Here's how the part is built. I have some questions about the finished solid (model axes, mm). Round coordinates to 2 decimals unless told otherwise and drop trailing zeros. Order: outer loops, then holes, each group sorted by start corner. A loop starts at its lowest first (then second) coordinate and runs counter-clockwise, first axis right, second up. Notation, with made-up numbers: (35.25, 45) - (78.25, 45) arc R19 cw to (78.25, 58) - close; hole circle Ø9 at (31.5, -24.75). An arc over 180 degrees is marked (long way). Answer as a JSON object with one key per item and string values.
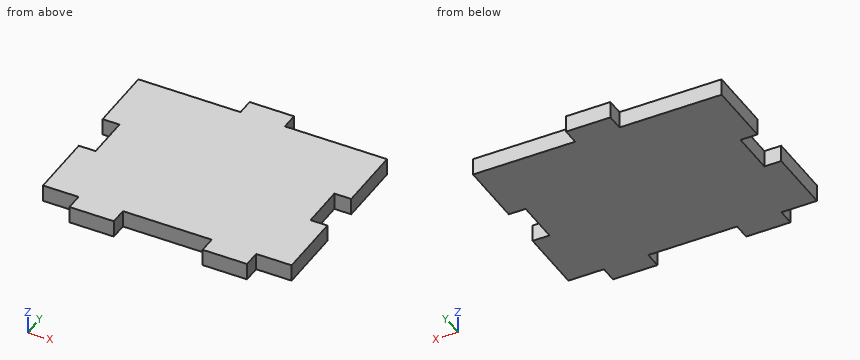
Autodesk Inventor part; units mm, degrees
ref_plane "YZ Plane" through (0, 0, 0) normal (1, 0, 0) x (0, 1, 0)
ref_plane "XZ Plane" through (0, 0, 0) normal (0, 1, 0) x (-1, 0, 0)
ref_plane "XY Plane" through (0, 0, 0) normal (0, 0, 1) x (1, 0, 0)
sketch "Sketch1" plane through (0, 0, 0) normal (0, 0, 1) x (1, 0, 0)
  line L0 (-34.925, 0) -> (34.925, 0)
  line L1 (-34.925, 4.826) -> (34.925, 4.826)
  line L2 (-25.4, 0) -> (-12.7, 0)
  line L3 (-25.4, 0) -> (-25.4, 4.826)
  line L4 (-12.7, 4.826) -> (-25.4, 4.826)
  line L5 (-12.7, 0) -> (-12.7, 4.826)
  line L6 (12.7, 0) -> (25.4, 0)
  line L7 (12.7, 0) -> (12.7, 4.826)
  line L8 (25.4, 4.826) -> (12.7, 4.826)
  line L9 (25.4, 0) -> (25.4, 4.826)
  line L10 (-34.925, 0) -> (-34.925, 4.826)
  line L11 (34.925, 4.826) -> (34.925, 0)
  point P0 (0, 0)
ref_plane "Work Plane1" through (-12.7, 0, -7.366) normal (0, 0, 1) x (1, 0, 0)
sketch "Sketch2" plane through (-12.7, 0, -7.366) normal (0, 0, 1) x (1, 0, 0)
  line L0 (0, 0) -> (-12.7, 0)
  line L1 (0, 0) -> (0, 4.826)
  line L2 (-12.7, 4.826) -> (0, 4.826)
  line L3 (-12.7, 0) -> (-12.7, 4.826)
  line L4 (-12.7, 0) -> (0, 0)
  line L5 (0, 0) -> (0, 4.826)
  line L6 (-12.7, 4.826) -> (-12.7, 0)
  line L7 (38.1, 0) -> (25.4, 0)
  line L8 (38.1, 0) -> (38.1, 4.826)
  line L9 (25.4, 4.826) -> (38.1, 4.826)
  line L10 (25.4, 0) -> (25.4, 4.826)
  line L11 (25.4, 0) -> (38.1, 0)
  line L12 (38.1, 0) -> (38.1, 4.826)
  line L13 (25.4, 4.826) -> (25.4, 0)
  line L14 (-18.034, 0) -> (-22.86, 0)
  line L15 (-18.034, 0) -> (-18.034, 4.826)
  line L16 (-22.86, 4.826) -> (-18.034, 4.826)
  line L17 (-22.86, 0) -> (-22.86, 4.826)
  line L18 (43.434, 0) -> (48.26, 0)
  line L19 (43.434, 0) -> (43.434, 4.826)
  line L20 (48.26, 4.826) -> (43.434, 4.826)
  line L21 (48.26, 0) -> (48.26, 4.826)
  line L22 (48.26, 55.626) -> (-22.86, 55.626)
  line L23 (-22.86, 36.576) -> (-18.034, 36.576)
  line L24 (-18.034, 36.576) -> (-18.034, 23.876)
  line L25 (-18.034, 23.876) -> (-22.86, 23.876)
  line L26 (48.26, 36.576) -> (43.434, 36.576)
  line L27 (43.434, 36.576) -> (43.434, 23.876)
  line L28 (43.434, 23.876) -> (48.26, 23.876)
  line L29 (-22.86, 55.626) -> (-22.86, 36.576)
  line L30 (-22.86, 23.876) -> (-22.86, 4.826)
  line L31 (48.26, 4.826) -> (48.26, 23.876)
  line L32 (48.26, 36.576) -> (48.26, 55.626)
  line L33 (-22.86, 4.826) -> (-12.7, 4.826)
  line L34 (0, 4.826) -> (25.4, 4.826)
  line L35 (38.1, 4.826) -> (48.26, 4.826)
  point P0 (12.7, 0)
  dimension "d0" = 50.8
  dimension "d2" = 12.7
  dimension "d5" = 4.826
  dimension "d13" = 19.05
  dimension "d14" = 19.05
  dimension "d15" = 12.7
extrude "Extrusion1" add sketch "Sketch2" along normal blind 4.826 contours L0 L3 L2 L1 | L2 L33 L16 L30 L25 L24 L23 L29 L22 L32 L26 L27 L28 L31 L20 L35 L9 L34 | L9 L8 L7 L10
sketch "Sketch3" plane through (-12.7, 0, -2.54) normal (0, 0, 1) x (1, 0, 0)
  line L0 (48.26, 55.626) -> (-22.86, 55.626)
  line L1 (-22.86, 55.626) -> (-22.86, 36.576)
  line L2 (48.26, 55.626) -> (-22.86, 55.626)
  line L3 (6.35, 55.626) -> (19.05, 55.626)
  line L4 (19.05, 55.626) -> (19.05, 60.452)
  line L5 (19.05, 60.452) -> (6.35, 60.452)
  line L6 (6.35, 60.452) -> (6.35, 55.626)
  point P0 (12.7, 0)
  dimension "d8" = 12.7
  dimension "d9" = 4.826
  dimension "d10" = 29.21
extrude "Extrusion2" add sketch "Sketch3" against normal blind 4.826
properties part number "sideL"
1. Imagine slicing it at B-B (x = -15.5). List the corners of the cut face in (y, z) for me.
Responses:
{"outline": "(0, -7.37) - (55.63, -7.37) - (55.63, -2.54) - (0, -2.54) - close"}
2. Imagine slicing it at C-C (y = 34.5). List the corners of the cut face in (x, z) for me.
Responses:
{"outline": "(-30.73, -7.37) - (30.73, -7.37) - (30.73, -2.54) - (-30.73, -2.54) - close"}
3. If I drill on L1, parallel to X at y = 4.5, z = -4.7; L2, parallel to Y at x = -17, z = -4.45; L3, parallel to X at y = 25, z = -4.75, over which ranges is the centre line in solid material (lowest first)? Write a range as [from, to].
Responses:
{"L1": "[-25.4, -12.7], [12.7, 25.4]", "L2": "[0, 55.63]", "L3": "[-30.73, 30.73]"}
4. For P1, Ø1.4, axis at y = 58.5, z = -5, coming from the +X side; P2, Ø2.5, axis at y = 2, z = -6, coming from the -X side; P3, Ø2.5, axis at y = 1.5, z = -4.5, coming from the +X side, each with a flat end and sliding along its axis, tell me the tip position at first contact or that it passes through.
Responses:
{"P1": "x = 6.35", "P2": "x = -25.4", "P3": "x = 25.4"}
5. Imagine slicing it at A-A (z = -6.25). List the corners of the cut face in (x, y) for me.
Responses:
{"outline": "(-35.56, 4.83) - (-25.4, 4.83) - (-25.4, 0) - (-12.7, 0) - (-12.7, 4.83) - (12.7, 4.83) - (12.7, 0) - (25.4, 0) - (25.4, 4.83) - (35.56, 4.83) - (35.56, 23.88) - (30.73, 23.88) - (30.73, 36.58) - (35.56, 36.58) - (35.56, 55.63) - (6.35, 55.63) - (6.35, 60.45) - (-6.35, 60.45) - (-6.35, 55.63) - (-35.56, 55.63) - (-35.56, 36.58) - (-30.73, 36.58) - (-30.73, 23.88) - (-35.56, 23.88) - close"}
